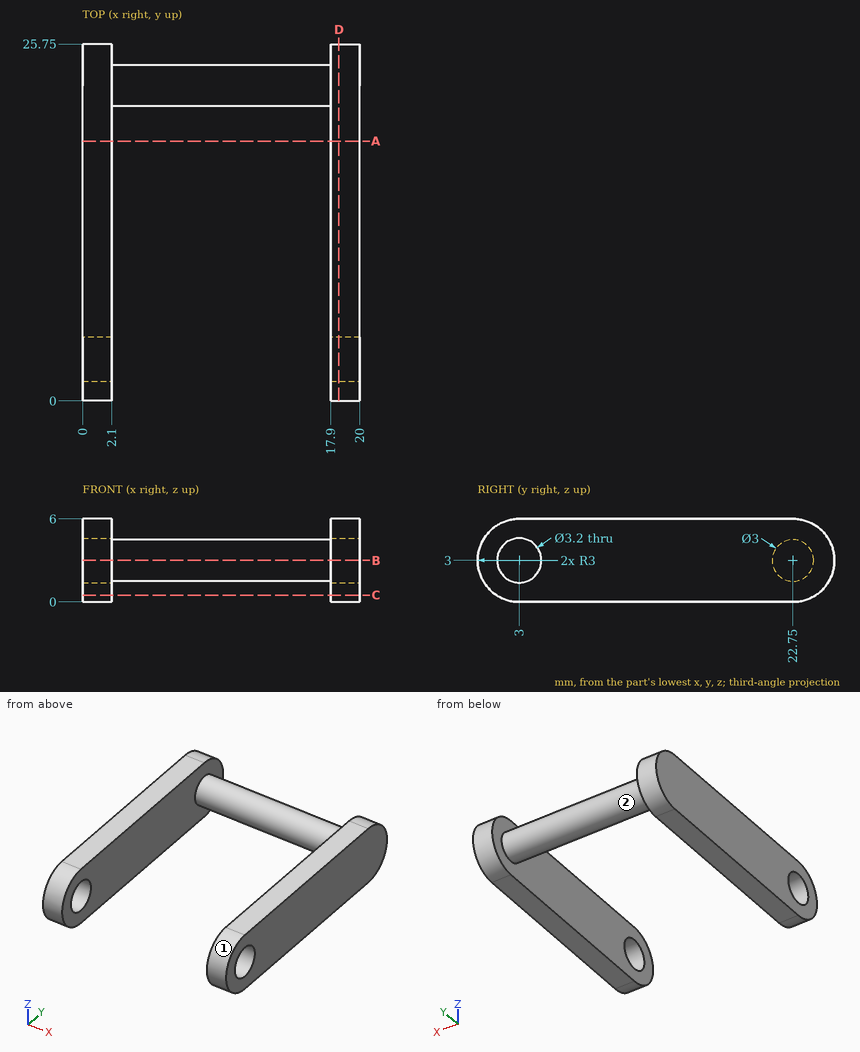
The drawing under review shows one solid part. Ordinate dimensions are in mm from its lowest x, y, z. A direction names the side the tool comes from. Coordinates: 2 decimals unless noted, no trailing zeros. Order: outer loops, then holes, each group sorted by start corner. A loop starts at its lowest first (then second) coordinate and runs counter-clockwise, first axis right, second up. Notation, with made-up numbers: (62.25, 63) -> (105.25, 63) arc R9 cw to (105.25, 68) -> close; hole circle Ø10 at (63, -10.5). An arc over 180 degrees is marked (long way). Return JSON: item names as keys, results as strings.
1. We need section A-A on y = 18.75. Write out the cut boundary in (x, z), and give its area (3 significant figures).
Answer block:
{"outline": "(0, 0) -> (2.1, 0) -> (2.1, 6) -> (0, 6) -> close; (17.9, 0) -> (20, 0) -> (20, 6) -> (17.9, 6) -> close", "area": "25.2 mm²"}
2. Machinability: for the marked faces 1 and 2, which of the approach directions +Z, -Z, +X, -X, +Y, -Y give a long, thin tool a straight path to every point of the face, cutting with its end or side? Answer none if there is none.
Answer block:
{"face 1": "+X, -X, -Y", "face 2": "none"}
3. For line 1 (Z direction, x = 0.6, y = 3); line 2 (X direction, y = 16.75, z = 3.75); line 3 (Y direction, x = 1.25, z = 3.5), list the stretches that pass through material, from the lowest coordinate up. Write a range as from..to.
Answer block:
{"line 1": "0..1.4, 4.6..6", "line 2": "0..2.1, 17.9..20", "line 3": "0.04..1.48, 4.52..25.71"}
4. For pin 1 Ø8 at (x, y) = (7, 16) entering from +Z; pin 2 Ø5 at (x, y) = (3.5, 15) entering from +Z, all flat-tipped, find the tip position at first contact; note any pin that passes through.
Answer block:
{"pin 1": "through", "pin 2": "z = 6"}
5. We need section B-B on z = 3. Write out the cut boundary in (x, y), and give its area (3 significant figures).
Answer block:
{"outline": "(0, 0) -> (2.1, 0) -> (2.1, 1.4) -> (0, 1.4) -> close; (0, 4.6) -> (2.1, 4.6) -> (2.1, 21.25) -> (17.9, 21.25) -> (17.9, 4.6) -> (20, 4.6) -> (20, 25.75) -> (17.9, 25.75) -> (17.9, 24.25) -> (2.1, 24.25) -> (2.1, 25.75) -> (0, 25.75) -> close; (17.9, 0) -> (20, 0) -> (20, 1.4) -> (17.9, 1.4) -> close", "area": "142 mm²"}
6. We need section D-D on x = 18.5. Write out the cut boundary in (y, z), and give its area (3 significant figures).
Answer block:
{"outline": "(3, 0) -> (22.75, 0) arc R3 ccw to (22.75, 6) -> (3, 6) arc R3 ccw to start; hole circle Ø3.2 at (3, 3)", "area": "139 mm²"}
7. We need section C-C on z = 0.5. Write out the cut boundary in (x, y).
Answer block:
{"outline": "(0, 1.34) -> (2.1, 1.34) -> (2.1, 24.41) -> (0, 24.41) -> close; (17.9, 1.34) -> (20, 1.34) -> (20, 24.41) -> (17.9, 24.41) -> close"}
